from build123d import *

# Parameters (mm, degrees)
F3_R      = 4
F3_R_2    = 12.5
F7_DEPTH  = 25
F4_R      = 12.5
F8_DEPTH  = 10
F5_R      = 17.5
F9_DEPTH  = 5
F6_R      = 6
F10_DEPTH = 5
F11_SIZE  = 1
F12_R     = 2


with BuildPart() as f7:
    # F3 (on Top) → F7 (new body)
    with BuildSketch(Plane.XY):
        with BuildLine():
            Line((30, 40), (-30, 40))
            ThreePointArc((-30, 40), (-37.071068, 37.071068), (-40, 30))
            Line((-40, 30), (-40, -30))
            ThreePointArc((-40, -30), (-37.071068, -37.071068), (-30, -40))
            Line((-30, -40), (30, -40))
            ThreePointArc((30, -40), (37.071068, -37.071068), (40, -30))
            Line((40, -30), (40, 30))
            ThreePointArc((40, 30), (37.071068, 37.071068), (30, 40))
        make_face()
        with Locations((-25, -25)):
            Circle(F3_R, mode=Mode.SUBTRACT)
        with Locations((25, -25)):
            Circle(F3_R, mode=Mode.SUBTRACT)
        with Locations((-25, 25)):
            Circle(F3_R, mode=Mode.SUBTRACT)
        Circle(F3_R_2, mode=Mode.SUBTRACT)
        with Locations((25, 25)):
            Circle(F3_R, mode=Mode.SUBTRACT)
    extrude(amount=F7_DEPTH)

    # F4 (on offset) → F8 (join)
    with BuildSketch(Plane.XY.offset(25)):
        with BuildLine():
            Line((15, 25), (-15, 25))
            ThreePointArc((-15, 25), (-17.928932, 17.928932), (-25, 15))
            Line((-25, 15), (-25, -15))
            ThreePointArc((-25, -15), (-17.928932, -17.928932), (-15, -25))
            Line((-15, -25), (15, -25))
            ThreePointArc((15, -25), (17.928932, -17.928932), (25, -15))
            Line((25, -15), (25, 15))
            ThreePointArc((25, 15), (17.928932, 17.928932), (15, 25))
        make_face()
        Circle(F4_R, mode=Mode.SUBTRACT)
    extrude(amount=F8_DEPTH)

    # F5 (on offset) → F9 (cut)
    with BuildSketch(Plane.XY.offset(30)):
        Circle(F5_R)
    extrude(amount=F9_DEPTH, mode=Mode.SUBTRACT)

    # F6 (on offset) → F10 (cut)
    with BuildSketch(Plane.XY.offset(20)):
        with Locations((-25, 25)):
            Circle(F6_R)
        with Locations((25, 25)):
            Circle(F6_R)
        with Locations((25, -25)):
            Circle(F6_R)
        with Locations((-25, -25)):
            Circle(F6_R)
    extrude(amount=F10_DEPTH, mode=Mode.SUBTRACT)

    # F11
    f11_edges = [f7.edges().sort_by_distance(p)[0] for p in [
        (-17.928932, 17.928932, 35),
        (-25, 0, 35),
        (-17.928932, -17.928932, 35),
        (0, -25, 35),
        (17.928932, -17.928932, 35),
        (25, 0, 35),
        (17.928932, 17.928932, 35),
        (0, 25, 35),
    ]]
    chamfer(f11_edges, length=F11_SIZE)

    # F12
    f12_edges = [f7.edges().sort_by_distance(p)[0] for p in [
        (-37.071068, -37.071068, 25),
        (-40, 0, 25),
    ]]
    fillet(f12_edges, radius=F12_R)


solid = f7.part
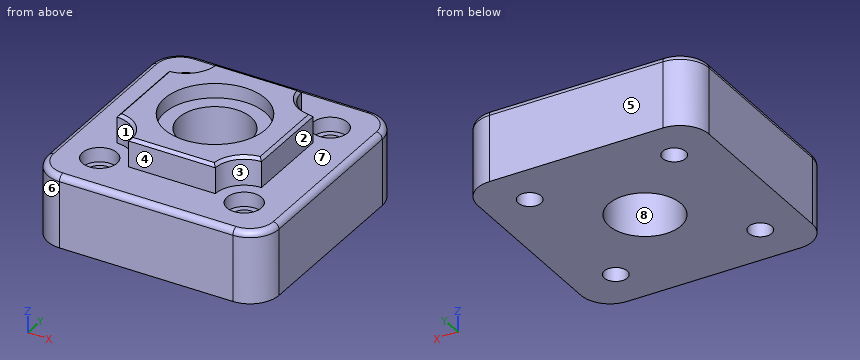
For this review, take the finished solid that the model builds, in its own axes (mm). Face numbers are marked on the shaded views. A direction names the side the tool comes from. Round coordinates to 2 decimals unless told otherwise and drop trailing zeros. Order: outer loops, then holes, each group sorted by start corner. A loop starts at its lowest first (then second) coordinate and runs counter-clockwise, first axis right, second up. Notation, with made-up numbers: M -13.5,37 L 4.5,37 A21 cw 4.5,72 Z; hole C 71.25,51.5 d10. An arc over 180 degrees is marked long. Write each question's results on one line, items separated by ' | '. Start each with the question number.
1. Add section A-A (x = 0). State the section outline as (y, z) points, then the cut area to 3 significant figures.
2. Clearance check with flat-ended pins moving along their axes: pin 1 Ø19 at (x, y) = (25, -25) entering from +Z; pin 2 Ø3 at (y, z) = (9, 25.5) entering from +X; pin 3 Ø9.5 at (x, y) = (25, 25) entering from +Z. State where each tip first meets the part, or that it passes through.
3. Add section C-C (z = 22). State the section outline as (x, y) points.
4. Draft analysis for pull direction Y (two halves, no side actions). For the marked faces 5, 6, 7 and 8, state which applies: pulls with the +Y half, pulls with the -Y half, needs draft (parallel to the pull), parting line crosses it, or undercut.
5. Add section D-D (y = -26.5). State the section outline as (x, z) points.
6. To check wall thickness, follow L1, parallel to Y at x = -25, z = 11; L2, parallel to Y at x = 25, z = 22.25; L3, parallel to X at y = 0, z = 9. State the ranges of each line that lie inside material, in increasing order. Write a range as [from, to].
7. Tool access review of the marked faces 1, 2, 3 and 4: name each direction out of +Z, -Z, +X, -X, +Y, -Y from which nothing blocks a thin tool from reaching the whole face with its end or side.
Output values:
1) outline: M -40,0 L -12.5,0 L -12.5,30 L -17.5,30 L -17.5,35 L -24,35 L -25,34 L -25,25 L -38,25 A2 ccw -40,23 Z; M 12.5,0 L 40,0 L 40,23 A2 ccw 38,25 L 25,25 L 25,34 L 24,35 L 17.5,35 L 17.5,30 L 12.5,30 Z | area: 1,570 mm^2
2) pin 1: z = 25 | pin 2: x = 39.73 | pin 3: z = 20
3) outline: M -40,-30 A10 ccw -30,-40 L 30,-40 A10 ccw 40,-30 L 40,30 A10 ccw 30,40 L -30,40 A10 ccw -40,30 Z; hole C -25,-25 d12; hole C -25,25 d12; hole C 0,0 d25; hole C 25,-25 d12; hole C 25,25 d12
4) face 5: pulls with the +Y half | face 6: pulls with the -Y half | face 7: needs draft | face 8: undercut
5) outline: M -40,0 L -28.71,0 L -28.71,20 L -30.81,20 L -30.81,25 L -38,25 A2 ccw -40,23 Z; M -21.29,0 L 21.29,0 L 21.29,20 L 19.19,20 L 19.19,25 L -19.19,25 L -19.19,20 L -21.29,20 Z; M 28.71,0 L 40,0 L 40,23 A2 ccw 38,25 L 30.81,25 L 30.81,20 L 28.71,20 Z
6) L1: [-40, -29], [-21, 21], [29, 40] | L2: [-40, -31], [-19, 19], [31, 40] | L3: [-40, -12.5], [12.5, 40]
7) face 1: +Z, -X, -Y | face 2: +Z, +X, +Y, -Y | face 3: +Z, +X, -Y | face 4: +Z, +X, -X, -Y
